from build123d import *

# Parameters (mm, degrees)
SKETCH3_R             = 2.35
BOSS_EXTRUDE1_DEPTH   = 3
BOSS_EXTRUDE1_2_DEPTH = 3
SKETCH3_W             = 4.6228
SKETCH3_H             = 4.6228
BOSS_EXTRUDE1_3_DEPTH = 3
BOSS_EXTRUDE1_4_DEPTH = 3
SKETCH4_R             = 7.5
SKETCH4_R_2           = 2.35
SKETCH4_W             = 25.4
SKETCH4_H             = 25.4
BOSS_EXTRUDE2_DEPTH   = 6
BOSS_EXTRUDE3_DEPTH   = 6.75
SKETCH7_R             = 2.35
CUT_EXTRUDE2_DEPTH    = 224.153476458
FILLET1_R             = 8
FILLET2_R             = 2.5
FILLET3_R             = 1.5
FILLET4_R             = 0.75


with BuildPart() as part:
    # Sketch3 → Boss-Extrude1 (new body)
    with BuildSketch(Plane.XY):
        with Locations((88.913961031, 184.15)):
            Circle(SKETCH3_R)
    extrude(amount=BOSS_EXTRUDE1_DEPTH)


with BuildPart() as body_2:
    # Sketch3 → Boss-Extrude1 2 (new body)
    with BuildSketch(Plane.XY):
        with Locations((76.213961031, 171.45)):
            Circle(SKETCH3_R)
    extrude(amount=BOSS_EXTRUDE1_2_DEPTH)


with BuildPart() as body_3:
    # Sketch3 → Boss-Extrude1 3 (new body)
    with BuildSketch(Plane.XY):
        with Locations((76.213961031, 184.15)):
            Rectangle(SKETCH3_W, SKETCH3_H)
    extrude(amount=BOSS_EXTRUDE1_3_DEPTH)



with BuildPart() as body_4:
    # Sketch3 → Boss-Extrude1 4 (new body)
    with BuildSketch(Plane.XY):
        with Locations((88.913961031, 171.45)):
            Rectangle(SKETCH3_W, SKETCH3_H)
    extrude(amount=BOSS_EXTRUDE1_4_DEPTH)


with BuildPart() as body_3_1:
    add(body_3.part)

    add(body_4.part)  # Boss-Extrude2 merges body 4

    add(body_2.part)  # Boss-Extrude2 merges body 2
    # Sketch4 → Boss-Extrude2 (add)
    # profile 1 of 2: a face of its own
    with BuildSketch(Plane(origin=(0, 0, 0), x_dir=(-1, 0, 0), z_dir=(0, 0, -1))):
        with Locations((-66.681980515, 193.681980515)):
            Circle(SKETCH4_R)
        with Locations((-66.681980515, 193.681980515)):
            Circle(SKETCH4_R_2, mode=Mode.SUBTRACT)
    # profile 2 of 2: a face of its own
    with BuildSketch(Plane(origin=(0, 0, 0), x_dir=(-1, 0, 0), z_dir=(0, 0, -1))):
        with Locations((-82.563961031, 177.8)):
            Rectangle(SKETCH4_W, SKETCH4_H)
    extrude(amount=BOSS_EXTRUDE2_DEPTH)

    # Sketch6 → Boss-Extrude3 (add)
    with BuildSketch(Plane(origin=(0, 0, -6), x_dir=(-1, 0, 0), z_dir=(0, 0, -1))):
        with BuildLine():
            Line((-73.748627528, 190.5), (-95.263961031, 190.5))
            Line((-95.263961031, 190.5), (-95.263961031, 165.1))
            Line((-95.263961031, 165.1), (-69.863961031, 165.1))
            Line((-69.863961031, 165.1), (-69.863961031, 186.615333503))
            ThreePointArc((-69.863961031, 186.615333503), (-72.16205807, 188.201902961), (-73.748627528, 190.5))
        make_face()
    extrude(amount=BOSS_EXTRUDE3_DEPTH)


with BuildPart() as cut_extrude2_tool:
    # Sketch7 → Cut-Extrude2 (new, through all)
    with BuildSketch(Plane.XY.offset(3)):
        with Locations((88.913961031, 184.15)):
            Circle(SKETCH7_R)
        with Locations((76.213961031, 171.45)):
            Circle(SKETCH7_R)
    extrude(amount=-CUT_EXTRUDE2_DEPTH)


with BuildPart() as part_1:
    add(part.part)

    # Cut-Extrude2: cut by cut_extrude2_tool
    add(cut_extrude2_tool.part, mode=Mode.SUBTRACT)


with BuildPart() as body_3_2:
    add(body_3_1.part)

    # Cut-Extrude2: cut by cut_extrude2_tool
    add(cut_extrude2_tool.part, mode=Mode.SUBTRACT)

    # Fillet1
    fillet1_edges = [body_3_2.edges().sort_by_distance(p)[0] for p in [
        (73.473519369, 190.5, -3),
    ]]
    fillet(fillet1_edges, radius=FILLET1_R)

    # Fillet2
    # the kernel refuses this fillet: 2.5 mm, written as the material it adds along each edge
    with BuildSketch(Plane(origin=(69.863961031, 186.890441662, -13.962947932), x_dir=(-0.9681157623464371, -0.25050323490202075, 0), z_dir=(0, 0, 1))) as fillet2_piece_1_section:
        with BuildLine():
            CenterArc((3.218187092, 2.457364076), FILLET2_R, 165.492706976, 93.910495797)
            Line((0.797897687, 3.083622163), (0, 0))
            ThreePointArc((0, 0), (1.37922304, 0.127907773), (2.758446079, 0))
        make_face()
    fillet2_piece_1 = extrude(amount=13.962947932, mode=Mode.PRIVATE)
    fillet2_piece_1 = split(fillet2_piece_1, bisect_by=Plane(origin=(69.434424627, 185.67157625, -6), z_dir=(0, 0, -1)), keep=Keep.TOP, mode=Mode.PRIVATE)
    fillet2_piece_1 = fillet2_piece_1 - Plane(origin=(66.681980515, 193.681980515, -9.375), x_dir=(0.4105781310115351, -0.9118254209743633, 0), z_dir=(0, 0, 1)) * Cylinder(7.75, 41, mode=Mode.PRIVATE)
    fillet2_piece_1 = split(fillet2_piece_1, bisect_by=Plane(origin=(69.434424627, 185.67157625, -12.75), z_dir=(0, 0, 1)), keep=Keep.TOP, mode=Mode.PRIVATE)
    add(fillet2_piece_1)
    with BuildSketch(Plane(origin=(69.863961031, 186.890441662, -6), x_dir=(-0.9681157623464371, -0.25050323490202075, 0), z_dir=(0, 0, 1))) as fillet2_piece_2_section:
        with BuildLine():
            CenterArc((3.218187092, 2.457364076), FILLET2_R, 165.492706976, 93.910495797)
            Line((0.797897687, 3.083622163), (0, 0))
            ThreePointArc((0, 0), (1.37922304, 0.127907773), (2.758446079, 0))
        make_face()
    fillet2_piece_2 = extrude(amount=6, mode=Mode.PRIVATE)
    fillet2_piece_2 = fillet2_piece_2 & Plane(origin=(66.681980515, 193.681980515, -3), x_dir=(0.4105781310115351, -0.9118254209743633, 0), z_dir=(0, 0, 1)) * Cylinder(7.75, 25, mode=Mode.PRIVATE)
    add(fillet2_piece_2)
    with BuildSketch(Plane(origin=(69.863961031, 186.890441662, -6), x_dir=(-0.9681157623464371, -0.25050323490202075, 0), z_dir=(0, 0, 1))) as fillet2_piece_3_section:
        with BuildLine():
            CenterArc((3.218187092, 2.457364076), FILLET2_R, 165.492706976, 93.910495797)
            Line((0.797897687, 3.083622163), (0, 0))
            ThreePointArc((0, 0), (1.37922304, 0.127907773), (2.758446079, 0))
        make_face()
    fillet2_piece_3 = extrude(amount=6, mode=Mode.PRIVATE)
    fillet2_piece_3 = fillet2_piece_3 - Plane(origin=(66.681980515, 193.681980515, -3), x_dir=(0.4105781310115351, -0.9118254209743633, 0), z_dir=(0, 0, 1)) * Cylinder(7.75, 25, mode=Mode.PRIVATE)
    add(fillet2_piece_3)

    # Fillet3
    fillet3_edges = [body_3_2.edges().sort_by_distance(p)[0] for p in [
        (74.361694574, 194.723369962, -9.375),
    ]]
    fillet(fillet3_edges, radius=FILLET3_R)

    # Fillet4
    fillet4_edges = [body_3_2.edges().sort_by_distance(p)[0] for p in [
        (91.225361031, 173.7614, 1.5),
        (86.602561031, 173.7614, 1.5),
        (86.602561031, 169.1386, 1.5),
        (91.225361031, 169.1386, 1.5),
        (78.525361031, 181.8386, 1.5),
        (73.902561031, 181.8386, 1.5),
        (73.902561031, 186.4614, 1.5),
        (78.525361031, 186.4614, 1.5),
    ]]
    fillet(fillet4_edges, radius=FILLET4_R)


solid = body_3_2.part
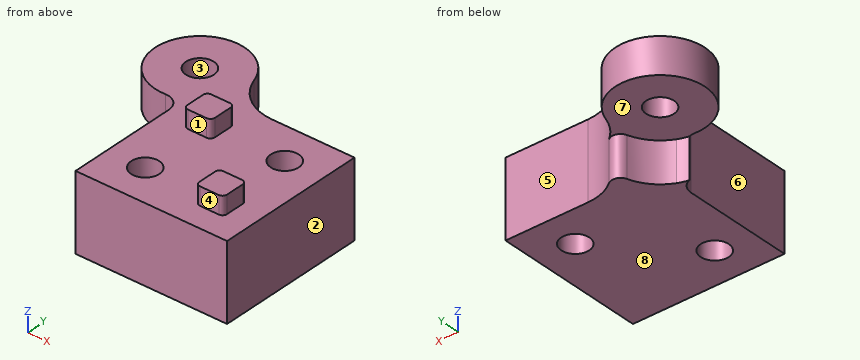
Check sheet for the modelled part. Datum: model origin and axes. Units: mm. Face numbers are marked on the shaded views. A direction names the side the tool comes from. Give positions to 0.01 mm unless a question says otherwise; leave off trailing zeros. Write each loop counter-clockwise with the first axis right and the second up, starting at its lowest first coordinate (ties: lowest second). Pieces come first, ordered by that corner, then holes. Notation, with made-up numbers: M 3,-17 L 52,-17 A8 ccw 52,-2 Z; hole C -31.75,-36.5 d7. An arc over 180 degrees is marked long. Use one line per item in the form item = value.
(1) Tool access check on the marked faces 4, 5, 6, 7 and 8. Record the directions out of +Z, -Z, +X, -X, +Y, -Y that give a thin tool (end or side, any length) a straight path to the whole face; none if there is none.
Answer block:
face_4 = +Z, +X, -X, -Y
face_5 = +Z, -Z, +X, +Y
face_6 = +Z, -Z, -X, -Y
face_7 = -Z, -X, +Y
face_8 = -Z, +X, -X, +Y, -Y
(2) Draft check along X on the marked faces 1, 2 and 3. Enter one of: pulls with the +X half, pulls with the -X half, needs draft (parallel to the pull), parting line crosses it, or undercut.
Answer block:
face_1 = needs draft
face_2 = pulls with the +X half
face_3 = undercut
(3) Section check D-D on y = 189.5. Record the boundary of the cut face in (x, z), plus the area to 3 significant figures.
Answer block:
outline = M 60.46,-6 L 73.21,-6 L 73.21,-12.75 L 95.26,-12.75 L 95.26,0 L 60.46,0 Z
area = 358 mm2
(4) Material ranges on line 1 along X through (y, z) = (171, -11); line 2 along Z through (x, y) = (93, 179.5); line 3 along Y through (x, z) = (87, -7.5), recorded low to high.
Answer block:
line_1 = 69.86 to 73.91, 78.52 to 95.26
line_2 = -12.75 to 0
line_3 = 165.1 to 182.79, 185.51 to 190.5
(5) Section check C-C on z = -1.75. Record the boundary of the cut face in (x, y), plus the area to 3 significant figures.
Answer block:
outline = M 67.19,186.2 A2.5 cw 69.86,183.71 L 69.86,165.1 L 95.26,165.1 L 95.26,190.5 L 81.41,190.5 A8 cw 73.81,196.01 A7.5 ccw long Z; hole C 66.68,193.68 d4.7; hole C 76.21,171.45 d4.7; hole C 88.91,184.15 d4.7
area = 774 mm2
(6) Section check B-B on x = 88.5. Record the boundary of the cut face in (y, z).
Answer block:
outline = M 165.1,-12.75 L 181.84,-12.75 L 181.84,0 L 173.76,0 L 173.76,3 L 169.14,3 L 169.14,0 L 165.1,0 Z; M 186.46,-12.75 L 190.5,-12.75 L 190.5,0 L 186.46,0 Z
(7) Section check A-A on y = 171.45. Record the boundary of the cut face in (x, z).
Answer block:
outline = M 69.86,-12.75 L 73.86,-12.75 L 73.86,0 L 69.86,0 Z; M 78.56,-12.75 L 95.26,-12.75 L 95.26,0 L 91.23,0 L 91.23,3 L 86.6,3 L 86.6,0 L 78.56,0 Z
(8) Depth check by flat-ended pin: P1, Ø12, axis at x = 64.5, y = 196.5, coming from the -Z side; P2, Ø0.9, axis at y = 171, z = 1, coming from the +X side; P3, Ø5, axis at y = 190, z = -3, coming from the -X side. Enter the tip coordinate at first touch or a pass-through.
Answer block:
P1 = -6
P2 = 91.23
P3 = 59.28
